```python
from build123d import *

# Parameters (mm, degrees)
SKETCH_1_W             = 295
SKETCH_1_H             = 65
SKETCH_1_R             = 2.5
EXTRUDE_1_DEPTH        = 3
SKETCH_4_R             = 5
CUT_EXTRUDE_2_DEPTH    = 15
SKETCH_6_R             = 2.1
CUT_EXTRUDE_4_DEPTH    = 10
SKETCH_7_R             = 7.5
SKETCH_7_R_2           = 5
CUT_EXTRUDE_5_DEPTH    = 10
FILLET_1_R             = 3
FILLET_2_R             = 5
EXTRUDE_3_DEPTH        = 3
EXTRUDE_4_DEPTH        = 3
SKETCH_10_R            = 7.5
EXTRUDE_5_DEPTH        = 3
SKETCH_12_R            = 2.498260172
SKETCH_12_R_2          = 2.5
EXTRUDE_6_DEPTH        = 3
SKETCH_14_R            = 7.5
EXTRUDE_7_DEPTH        = 3
SKETCH_16_R            = 2.5
CUT_EXTRUDE_9_DEPTH    = 4
FILLET_1_OF_MIRROR_4_R = 3
SKETCH_17_R            = 7.5
EXTRUDE_9_DEPTH        = 3
SKETCH_18_R            = 5
EXTRUDE_10_DEPTH       = 3
SKETCH_19_R            = 2.499999993
SKETCH_19_R_2          = 2.5
CUT_EXTRUDE_10_DEPTH   = 10


with BuildPart() as part:
    # 草图1 → 凸台-拉伸1 (new body)
    with BuildSketch(Plane(origin=(0, 0, 0), x_dir=(1, 0, 0), z_dir=(0, 1, 0))):
        Rectangle(SKETCH_1_W, SKETCH_1_H)
        with Locations((-137.5, 12.5)):
            Circle(SKETCH_1_R, mode=Mode.SUBTRACT)
        with Locations((-112.5, 12.5)):
            Circle(SKETCH_1_R, mode=Mode.SUBTRACT)
        with Locations((-137.5, -12.5)):
            Circle(SKETCH_1_R, mode=Mode.SUBTRACT)
        with Locations((-112.5, -12.5)):
            Circle(SKETCH_1_R, mode=Mode.SUBTRACT)
        with Locations((-20, 12)):
            Circle(SKETCH_1_R, mode=Mode.SUBTRACT)
        with Locations((-20, -12)):
            Circle(SKETCH_1_R, mode=Mode.SUBTRACT)
        with Locations((20, -12)):
            Circle(SKETCH_1_R, mode=Mode.SUBTRACT)
        with Locations((20, 12)):
            Circle(SKETCH_1_R, mode=Mode.SUBTRACT)
        with Locations((112.5, -12.5)):
            Circle(SKETCH_1_R, mode=Mode.SUBTRACT)
        with Locations((137.5, -12.5)):
            Circle(SKETCH_1_R, mode=Mode.SUBTRACT)
        with Locations((112.5, 12.5)):
            Circle(SKETCH_1_R, mode=Mode.SUBTRACT)
        with Locations((137.5, 12.5)):
            Circle(SKETCH_1_R, mode=Mode.SUBTRACT)
    extrude(amount=EXTRUDE_1_DEPTH)

    # 草图4 → 切除-拉伸2 (cut)
    with BuildSketch(Plane(origin=(0, 3, 0), x_dir=(1, 0, 0), z_dir=(0, 1, 0))):
        with Locations((112.5, -12.5)):
            Circle(SKETCH_4_R)
        with Locations((112.5, 12.5)):
            Circle(SKETCH_4_R)
        with Locations((137.5, -12.5)):
            Circle(SKETCH_4_R)
        with Locations((137.5, 12.5)):
            Circle(SKETCH_4_R)
        with Locations((-137.5, 12.5)):
            Circle(SKETCH_4_R)
        with Locations((-137.5, -12.5)):
            Circle(SKETCH_4_R)
        with Locations((-112.5, 12.5)):
            Circle(SKETCH_4_R)
        with Locations((-112.5, -12.5)):
            Circle(SKETCH_4_R)
    extrude(amount=-CUT_EXTRUDE_2_DEPTH, mode=Mode.SUBTRACT)

    # 草图6 → 切除-拉伸4 (cut)
    with BuildSketch(Plane(origin=(0, 3, 0), x_dir=(1, 0, 0), z_dir=(0, 1, 0))):
        with Locations((136, -25)):
            Circle(SKETCH_6_R)
        with Locations((-136, -25)):
            Circle(SKETCH_6_R)
        with Locations((-136, 25)):
            Circle(SKETCH_6_R)
        with Locations((136, 25)):
            Circle(SKETCH_6_R)
        with Locations((114, -25)):
            Circle(SKETCH_6_R)
        with Locations((-114, -25)):
            Circle(SKETCH_6_R)
        with Locations((114, 25)):
            Circle(SKETCH_6_R)
        with Locations((-114, 25)):
            Circle(SKETCH_6_R)
    extrude(amount=-CUT_EXTRUDE_4_DEPTH, mode=Mode.SUBTRACT)

    # 草图7 → 切除-拉伸5 (cut)
    with BuildSketch(Plane(origin=(0, 3, 0), x_dir=(1, 0, 0), z_dir=(0, 1, 0))):
        with Locations((-66.25, 19.5)):
            Circle(SKETCH_7_R)
        with Locations((-66.25, -19.5)):
            Circle(SKETCH_7_R)
        with Locations((66.25, 19.5)):
            Circle(SKETCH_7_R)
        with Locations((66.25, -19.5)):
            Circle(SKETCH_7_R)
        with Locations((-30, 22.5)):
            Circle(SKETCH_7_R_2)
        with Locations((-15, 22.5)):
            Circle(SKETCH_7_R_2)
        with Locations((15, 22.5)):
            Circle(SKETCH_7_R_2)
        with Locations((30, 22.5)):
            Circle(SKETCH_7_R_2)
        with Locations((-30, -22.5)):
            Circle(SKETCH_7_R_2)
        with Locations((-15, -22.5)):
            Circle(SKETCH_7_R_2)
        with Locations((15, -22.5)):
            Circle(SKETCH_7_R_2)
        with Locations((30, -22.5)):
            Circle(SKETCH_7_R_2)
        with Locations((0, 22.5)):
            Circle(SKETCH_7_R_2)
        with Locations((0, -22.5)):
            Circle(SKETCH_7_R_2)
        Polygon((-86.25, 27.5), (-102.5, 3.5), (-70, 3.5), align=None)
        Polygon((-30, 3.5), (-62.5, 3.5), (-46.25, 27.5), align=None)
        Polygon((-102.5, -3.5), (-70, -3.5), (-86.25, -27.5), align=None)
        Polygon((-46.25, -27.5), (-30, -3.5), (-62.5, -3.5), align=None)
        Polygon((46.25, 27.5), (30, 3.5), (62.5, 3.5), align=None)
        Polygon((102.5, 3.5), (70, 3.5), (86.25, 27.5), align=None)
        Polygon((86.25, -27.5), (102.5, -3.5), (70, -3.5), align=None)
        Polygon((62.5, -3.5), (46.25, -27.5), (30, -3.5), align=None)
    cut_extrude_5 = extrude(amount=-CUT_EXTRUDE_5_DEPTH, mode=Mode.SUBTRACT)

    # 圆角1
    fillet_1_edges = [part.edges().sort_by_distance(p)[0] for p in [
        (86.25, 1.5, -27.5),
        (102.5, 1.5, -3.5),
        (70, 1.5, -3.5),
        (86.25, 1.5, 27.5),
        (70, 1.5, 3.5),
        (102.5, 1.5, 3.5),
        (30, 1.5, 3.5),
        (62.5, 1.5, 3.5),
        (46.25, 1.5, 27.5),
        (-46.25, 1.5, -27.5),
        (-30, 1.5, -3.5),
        (-62.5, 1.5, -3.5),
        (-86.25, 1.5, 27.5),
        (-102.5, 1.5, 3.5),
        (-70, 1.5, 3.5),
        (46.25, 1.5, -27.5),
        (62.5, 1.5, -3.5),
        (30, 1.5, -3.5),
        (-46.25, 1.5, 27.5),
        (-62.5, 1.5, 3.5),
        (-30, 1.5, 3.5),
        (-86.25, 1.5, -27.5),
        (-70, 1.5, -3.5),
        (-102.5, 1.5, -3.5),
    ]]
    fillet(fillet_1_edges, radius=FILLET_1_R)

    # 圆角2
    fillet_2_edges = [part.edges().sort_by_distance(p)[0] for p in [
        (147.5, 1.5, 32.5),
        (-147.5, 1.5, 32.5),
        (-147.5, 1.5, -32.5),
        (147.5, 1.5, -32.5),
    ]]
    fillet(fillet_2_edges, radius=FILLET_2_R)

    # 草图8 → 凸台-拉伸3 (add)
    with BuildSketch(Plane.XZ):
        with BuildLine():
            Line((-88.734143599, 23.831110992), (-99.329914637, 8.181972229))
            ThreePointArc((-99.329914637, 8.181972229), (-99.495857516, 5.093926866), (-96.845771038, 3.5))
            Line((-96.845771038, 3.5), (-75.654228962, 3.5))
            ThreePointArc((-75.654228962, 3.5), (-73.004142484, 5.093926866), (-73.170085363, 8.181972229))
            Line((-73.170085363, 8.181972229), (-83.765856401, 23.831110992))
            ThreePointArc((-83.765856401, 23.831110992), (-86.25, 25.149138763), (-88.734143599, 23.831110992))
        make_face()
    extrude(amount=-EXTRUDE_3_DEPTH)

    # 草图9 → 凸台-拉伸4 (add)
    with BuildSketch(Plane.XZ):
        with BuildLine():
            Line((-88.734143599, -23.831110992), (-99.329914637, -8.181972229))
            ThreePointArc((-99.329914637, -8.181972229), (-99.495857516, -5.093926866), (-96.845771038, -3.5))
            Line((-96.845771038, -3.5), (-75.654228962, -3.5))
            ThreePointArc((-75.654228962, -3.5), (-73.004142484, -5.093926866), (-73.170085363, -8.181972229))
            Line((-73.170085363, -8.181972229), (-83.765856401, -23.831110992))
            ThreePointArc((-83.765856401, -23.831110992), (-86.25, -25.149138763), (-88.734143599, -23.831110992))
        make_face()
    extrude(amount=-EXTRUDE_4_DEPTH)

    # 草图10 → 凸台-拉伸5 (add)
    with BuildSketch(Plane.XZ):
        with Locations((-66.25, -19.5)):
            Circle(SKETCH_10_R)
        with Locations((-66.25, 19.5)):
            Circle(SKETCH_10_R)
    extrude(amount=-EXTRUDE_5_DEPTH)

    # 草图12 → 凸台-拉伸6 (add)
    with BuildSketch(Plane.XZ):
        with Locations((-20, -12)):
            Circle(SKETCH_12_R)
        with Locations((-20, 12)):
            Circle(SKETCH_12_R_2)
        with Locations((20, -12)):
            Circle(SKETCH_12_R_2)
        with Locations((20, 12)):
            Circle(SKETCH_12_R_2)
    extrude(amount=-EXTRUDE_6_DEPTH)

    # 草图14 → 凸台-拉伸7 (add)
    with BuildSketch(Plane.XZ):
        with Locations((66.25, -19.5)):
            Circle(SKETCH_14_R)
        with Locations((66.25, 19.5)):
            Circle(SKETCH_14_R)
    extrude(amount=-EXTRUDE_7_DEPTH)

    # 草图16 → 切除-拉伸9 (cut, through all)
    with BuildSketch(Plane(origin=(0, 3, 0), x_dir=(1, 0, 0), z_dir=(0, 1, 0))):
        with Locations((-20, -12)):
            Circle(SKETCH_16_R)
        with Locations((-20, 12)):
            Circle(SKETCH_16_R)
        with Locations((20, -12)):
            Circle(SKETCH_16_R)
        with Locations((20, 12)):
            Circle(SKETCH_16_R)
    extrude(amount=-CUT_EXTRUDE_9_DEPTH, mode=Mode.SUBTRACT)

    # 镜向4: 切除-拉伸5 across plane
    add(cut_extrude_5.mirror(Plane(origin=(0, 0, 0), x_dir=(0, 0, 1), z_dir=(1, 0, 0))), mode=Mode.SUBTRACT)

    # 圆角1 of 镜向4
    fillet_1_of_mirror_4_edges = [part.edges().sort_by_distance(p)[0] for p in [
        (-86.25, 1.5, -27.5),
        (-102.5, 1.5, -3.5),
        (-70, 1.5, -3.5),
        (-86.25, 1.5, 27.5),
        (-70, 1.5, 3.5),
        (-102.5, 1.5, 3.5),
        (-30, 1.5, 3.5),
        (-62.5, 1.5, 3.5),
        (-46.25, 1.5, 27.5),
        (46.25, 1.5, -27.5),
        (30, 1.5, -3.5),
        (62.5, 1.5, -3.5),
        (86.25, 1.5, 27.5),
        (102.5, 1.5, 3.5),
        (70, 1.5, 3.5),
        (-46.25, 1.5, -27.5),
        (-62.5, 1.5, -3.5),
        (-30, 1.5, -3.5),
        (46.25, 1.5, 27.5),
        (62.5, 1.5, 3.5),
        (30, 1.5, 3.5),
        (86.25, 1.5, -27.5),
        (70, 1.5, -3.5),
        (102.5, 1.5, -3.5),
    ]]
    fillet(fillet_1_of_mirror_4_edges, radius=FILLET_1_OF_MIRROR_4_R)

    # 草图17 → 凸台-拉伸9 (add)
    with BuildSketch(Plane(origin=(0, 3, 0), x_dir=(1, 0, 0), z_dir=(0, 1, 0))):
        with Locations((-66.25, 19.5)):
            Circle(SKETCH_17_R)
        with Locations((-66.25, -19.5)):
            Circle(SKETCH_17_R)
        with Locations((66.25, 19.5)):
            Circle(SKETCH_17_R)
        with Locations((66.25, -19.5)):
            Circle(SKETCH_17_R)
        with BuildLine():
            Line((-48.734143599, 23.831110992), (-59.329914637, 8.181972229))
            ThreePointArc((-59.329914637, 8.181972229), (-59.495857516, 5.093926866), (-56.845771038, 3.5))
            Line((-56.845771038, 3.5), (-35.654228962, 3.5))
            ThreePointArc((-35.654228962, 3.5), (-33.004142484, 5.093926866), (-33.170085363, 8.181972229))
            Line((-33.170085363, 8.181972229), (-43.765856401, 23.831110992))
            ThreePointArc((-43.765856401, 23.831110992), (-46.25, 25.149138763), (-48.734143599, 23.831110992))
        make_face()
        with BuildLine():
            Line((-56.845771038, -3.5), (-35.654228962, -3.5))
            ThreePointArc((-35.654228962, -3.5), (-33.004142484, -5.093926866), (-33.170085363, -8.181972229))
            Line((-33.170085363, -8.181972229), (-43.765856401, -23.831110992))
            ThreePointArc((-43.765856401, -23.831110992), (-46.25, -25.149138763), (-48.734143599, -23.831110992))
            Line((-48.734143599, -23.831110992), (-59.329914637, -8.181972229))
            ThreePointArc((-59.329914637, -8.181972229), (-59.495857516, -5.093926866), (-56.845771038, -3.5))
        make_face()
        with BuildLine():
            Line((43.765856401, 23.831110992), (33.170085363, 8.181972229))
            ThreePointArc((33.170085363, 8.181972229), (33.004142484, 5.093926866), (35.654228962, 3.5))
            Line((35.654228962, 3.5), (56.845771038, 3.5))
            ThreePointArc((56.845771038, 3.5), (59.495857516, 5.093926866), (59.329914637, 8.181972229))
            Line((59.329914637, 8.181972229), (48.734143599, 23.831110992))
            ThreePointArc((48.734143599, 23.831110992), (46.25, 25.149138763), (43.765856401, 23.831110992))
        make_face()
        with BuildLine():
            Line((35.654228962, -3.5), (56.845771038, -3.5))
            ThreePointArc((56.845771038, -3.5), (59.495857516, -5.093926866), (59.329914637, -8.181972229))
            Line((59.329914637, -8.181972229), (48.734143599, -23.831110992))
            ThreePointArc((48.734143599, -23.831110992), (46.25, -25.149138763), (43.765856401, -23.831110992))
            Line((43.765856401, -23.831110992), (33.170085363, -8.181972229))
            ThreePointArc((33.170085363, -8.181972229), (33.004142484, -5.093926866), (35.654228962, -3.5))
        make_face()
    extrude(amount=-EXTRUDE_9_DEPTH)

    # 草图18 → 凸台-拉伸10 (add)
    with BuildSketch(Plane.XZ):
        with Locations((-30, -22.5)):
            Circle(SKETCH_18_R)
        with Locations((30, -22.5)):
            Circle(SKETCH_18_R)
        with Locations((30, 22.5)):
            Circle(SKETCH_18_R)
        with Locations((-30, 22.5)):
            Circle(SKETCH_18_R)
    extrude(amount=-EXTRUDE_10_DEPTH)

    # 草图19 → 切除-拉伸10 (cut)
    with BuildSketch(Plane(origin=(0, 0, 0), x_dir=(-1, 0, 0), z_dir=(0, -1, 0))):
        with Locations((-33.500000037, 14.99999998)):
            Circle(SKETCH_19_R)
        with Locations((-33.500000051, 0)):
            Circle(SKETCH_19_R_2)
        with Locations((33.499999962, 14.937012041)):
            Circle(SKETCH_19_R_2)
        with Locations((33.499999962, -0.062987959)):
            Circle(SKETCH_19_R_2)
    extrude(amount=-CUT_EXTRUDE_10_DEPTH, mode=Mode.SUBTRACT)


solid = part.part
```
Could you check a few things on this model? Use its own coordinates, in mm. Round coordinates to 2 decimals unless told otherwise and drop trailing zeros. Loops run counter-clockwise (first coordinate to the right, second up) from the corner with the lowest first, then second, coordinate; pieces in that order, holes last. Notation, with made-up numbers: (67.25, 22) - (73.25, 22) arc R16 ccw to (73.25, 27) - close; hole circle Ø6 at (15, 73). An arc over 180 degrees is marked (long way). Answer in a Markdown table with one row per item. Add a question column.
(1) I need wall thicknesses on line 1 along Z through (x, y) = (15, 2.25); line 2 along X through (y, z) = (1.8, -7); line 3 along Z through (x, y) = (-33.5, 0.4). Which ranges of each line are inside material? Lowest first, please.
(2) If we section it at A-A (x = 33.5): Please give me the cut outline in (y, z), plus the area to 3 significant figures.
(3) If we mould it in two halves opening along Z, with no side actions, what happens to faces 1 (the face through (-2, 3, 0)), 2 (the face through (142.27, 1.52, -14)), 3 (the face through (-146.07, 1.52, 31))? For each: pulls with the +Z half, pulls with the -Z half, needs draft (parallel to the pull), parting line crosses it, or undercut.
(4) If we section it at B-B (y = 0.75): State how many separate pieces and enclosed holes the cut face has, plus the area to 3 significant figures.
Model answer:
| question | item | result |
|---|---|---|
| 1 | line 1 | z = -32.5 to -27.5, -17.5 to 17.5, 27.5 to 32.5 |
| 1 | line 2 | x = -147.5 to -99.8, -72.7 to 72.7, 99.8 to 147.5 |
| 1 | line 3 | z = -32.5 to -17.44, -12.44 to -2.44, 2.56 to 32.5 |
| 2 | outline | (0, -32.5) - (3, -32.5) - (3, -17.5) - (0, -17.5) - close; (0, -12.5) - (3, -12.5) - (3, -2.5) - (0, -2.5) - close; (0, 2.5) - (3, 2.5) - (3, 32.5) - (0, 32.5) - close |
| 2 | area | 165 mm² |
| 3 | face 1 | needs draft |
| 3 | face 2 | undercut |
| 3 | face 3 | pulls with the +Z half |
| 4 | separate pieces | 1 |
| 4 | enclosed holes | 34 |
| 4 | area | 16,300 mm² |
